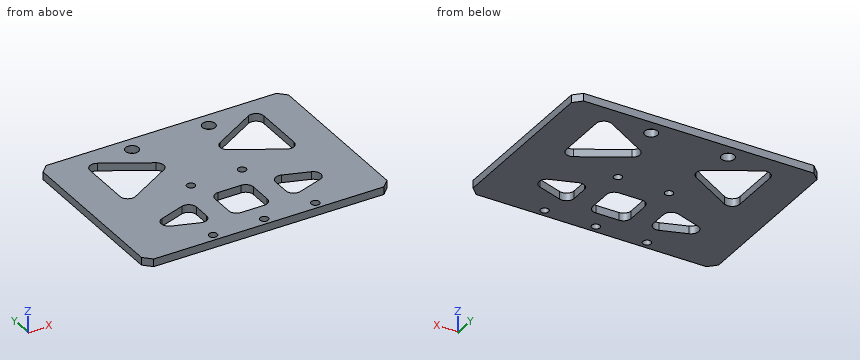
```python
from build123d import *

# Parameters (mm, degrees)
SKETCH_1_W           = 20
SKETCH_1_H           = 40
SKETCH_1_W_2         = 14
SKETCH_1_H_2         = 34
EXTRUDE_1_DEPTH      = 321
SKETCH_15_R          = 2.525
CUT_EXTRUDE_12_DEPTH = 21
SKETCH_18_W          = 17
SKETCH_18_H          = 40
CUT_EXTRUDE_14_DEPTH = 322
SKETCH_19_W          = 96
SKETCH_19_H          = 30
EXTRUDE_2_DEPTH      = 3
SKETCH_17_R          = 1.6
CUT_EXTRUDE_13_DEPTH = 4
FILLET_1_R           = 2
CHAMFER_1_SIZE       = 3
SKETCH_20_W          = 11
SKETCH_20_H          = 22.5
SKETCH_20_W_2        = 15
SKETCH_20_H_2        = 15
CUT_EXTRUDE_15_DEPTH = 4
FILLET_2_R           = 3
CUT_EXTRUDE_16_DEPTH = 4
FILLET_3_R           = 2
SKETCH_22_R          = 1.6
CUT_EXTRUDE_17_DEPTH = 4
CUT_EXTRUDE_19_DEPTH = 10
CHAMFER_2_SIZE       = 3
EXTRUDE_3_DEPTH      = 3
CUT_EXTRUDE_20_DEPTH = 4
FILLET_4_R           = 3


with BuildPart() as part:
    # 草图1 → 凸台-拉伸1 (new body)
    with BuildSketch(Plane(origin=(0, 0, 0), x_dir=(0, 0, -1), z_dir=(1, 0, 0))):
        Rectangle(SKETCH_1_W, SKETCH_1_H)
        Rectangle(SKETCH_1_W_2, SKETCH_1_H_2, mode=Mode.SUBTRACT)
    extrude(amount=EXTRUDE_1_DEPTH)

    # 草图15 → 切除-拉伸12 (cut, through all)
    with BuildSketch(Plane.XY.offset(10)):
        with Locations((145.5, 14)):
            Circle(SKETCH_15_R)
        with Locations((175.5, 14)):
            Circle(SKETCH_15_R)
    extrude(amount=-CUT_EXTRUDE_12_DEPTH, mode=Mode.SUBTRACT)

    # 草图18 → 切除-拉伸14 (cut, through all)
    with BuildSketch(Plane(origin=(321, 0, 0), x_dir=(0, 0, -1), z_dir=(1, 0, 0))):
        with Locations((1.5, 0)):
            Rectangle(SKETCH_18_W, SKETCH_18_H)
    extrude(amount=-CUT_EXTRUDE_14_DEPTH, mode=Mode.SUBTRACT)

    # 草图19 → 凸台-拉伸2 (add)
    with BuildSketch(Plane.XY.offset(10)):
        with Locations((160.5, -35)):
            Rectangle(SKETCH_19_W, SKETCH_19_H)
    extrude(amount=-EXTRUDE_2_DEPTH)

    # 草图17 → 切除-拉伸13 (cut, through all)
    with BuildSketch(Plane.XY.offset(10)):
        with Locations((12, 16.5)):
            Circle(SKETCH_17_R)
        with Locations((29, 16.5)):
            Circle(SKETCH_17_R)
        with Locations((12, -14)):
            Circle(SKETCH_17_R)
        with Locations((29, -14)):
            Circle(SKETCH_17_R)
        with Locations((43.5, -14)):
            Circle(SKETCH_17_R)
        with Locations((67.5, -14)):
            Circle(SKETCH_17_R)
        with Locations((222, -14)):
            Circle(SKETCH_17_R)
        with Locations((239, -14)):
            Circle(SKETCH_17_R)
        with Locations((253.5, -14)):
            Circle(SKETCH_17_R)
        with Locations((277.5, -14)):
            Circle(SKETCH_17_R)
        with Locations((292, -14)):
            Circle(SKETCH_17_R)
        with Locations((309, -14)):
            Circle(SKETCH_17_R)
        with Locations((82, -14)):
            Circle(SKETCH_17_R)
        with Locations((99, -14)):
            Circle(SKETCH_17_R)
        with Locations((292, 16.5)):
            Circle(SKETCH_17_R)
        with Locations((309, 16.5)):
            Circle(SKETCH_17_R)
        with Locations((140.5, -47)):
            Circle(SKETCH_17_R)
        with Locations((160.5, -47)):
            Circle(SKETCH_17_R)
        with Locations((180.5, -47)):
            Circle(SKETCH_17_R)
    extrude(amount=-CUT_EXTRUDE_13_DEPTH, mode=Mode.SUBTRACT)

    # 圆角1
    fillet_1_edges = [part.edges().sort_by_distance(p)[0] for p in [
        (208.5, -20, 8.5),
        (112.5, -20, 8.5),
    ]]
    fillet(fillet_1_edges, radius=FILLET_1_R)

    # 倒角1
    chamfer_1_edges = [part.edges().sort_by_distance(p)[0] for p in [
        (0, 20, 8.5),
        (321, 20, 8.5),
        (0, -20, 8.5),
        (208.5, -50, 8.5),
        (112.5, -50, 8.5),
        (321, -20, 8.5),
    ]]
    chamfer(chamfer_1_edges, length=CHAMFER_1_SIZE)

    # 草图20 → 切除-拉伸15 (cut, through all)
    with BuildSketch(Plane.XY.offset(10)):
        with Locations((300.5, 1.25)):
            Rectangle(SKETCH_20_W, SKETCH_20_H)
        with Locations((20.5, 1.25)):
            Rectangle(SKETCH_20_W, SKETCH_20_H)
        with Locations((160.5, -32)):
            Rectangle(SKETCH_20_W_2, SKETCH_20_H_2)
        Polygon((123, -32), (145, -24.5), (145, -39.5), align=None)
        Polygon((176, -24.5), (176, -39.5), (198, -32), align=None)
    extrude(amount=-CUT_EXTRUDE_15_DEPTH, mode=Mode.SUBTRACT)

    # 圆角2
    fillet_2_edges = [part.edges().sort_by_distance(p)[0] for p in [
        (26, 12.5, 8.5),
        (26, -10, 8.5),
        (15, -10, 8.5),
        (15, 12.5, 8.5),
        (176, -24.5, 8.5),
        (198, -32, 8.5),
        (176, -39.5, 8.5),
        (145, -39.5, 8.5),
        (123, -32, 8.5),
        (145, -24.5, 8.5),
        (168, -24.5, 8.5),
        (168, -39.5, 8.5),
        (153, -39.5, 8.5),
        (153, -24.5, 8.5),
        (306, 12.5, 8.5),
        (306, -10, 8.5),
        (295, -10, 8.5),
        (295, 12.5, 8.5),
    ]]
    fillet(fillet_2_edges, radius=FILLET_2_R)

    # 草图21 → 切除-拉伸16 (cut, through all)
    with BuildSketch(Plane.XY.offset(10)):
        Polygon((33, 6.144919815), (33, -10), (55.199264746, -10), align=None)
        Polygon((181.103828979, -10), (139.896171021, -10), (160.5, 8.609910045), align=None)
        Polygon((67.248892355, -8.871386982), (41.300735254, 10), (88.479202711, 10), align=None)
        Polygon((288, -10), (265.800735254, -10), (288, 6.144919815), align=None)
        Polygon((253.751107645, -8.871386982), (232.520797289, 10), (279.699264746, 10), align=None)
    extrude(amount=-CUT_EXTRUDE_16_DEPTH, mode=Mode.SUBTRACT)

    # 圆角3
    fillet_3_edges = [part.edges().sort_by_distance(p)[0] for p in [
        (279.699264746, 10, 8.5),
        (253.751107645, -8.871386982, 8.5),
        (232.520797289, 10, 8.5),
        (265.800735254, -10, 8.5),
        (288, 6.144919815, 8.5),
        (288, -10, 8.5),
        (160.5, 8.609910045, 8.5),
        (181.103828979, -10, 8.5),
        (139.896171021, -10, 8.5),
        (88.479202711, 10, 8.5),
        (67.248892355, -8.871386982, 8.5),
        (41.300735254, 10, 8.5),
        (33, 6.144919815, 8.5),
        (55.199264746, -10, 8.5),
        (33, -10, 8.5),
    ]]
    fillet(fillet_3_edges, radius=FILLET_3_R)

    # 草图22 → 切除-拉伸17 (cut, through all)
    with BuildSketch(Plane.XY.offset(10)):
        with Locations((150.5, -16)):
            Circle(SKETCH_22_R)
        with Locations((170.5, -16)):
            Circle(SKETCH_22_R)
    extrude(amount=-CUT_EXTRUDE_17_DEPTH, mode=Mode.SUBTRACT)

    # 草图26 → 切除-拉伸19 (cut)
    with BuildSketch(Plane.XY.offset(10)):
        with BuildLine():
            ThreePointArc((110.5, -20), (111.914213562, -20.585786438), (112.5, -22))
            Line((112.5, -22), (112.5, 20))
            Line((112.5, 20), (3, 20))
            Line((3, 20), (0, 17))
            Line((0, 17), (0, -17))
            Line((0, -17), (3, -20))
            Line((3, -20), (110.5, -20))
        make_face()
        with BuildLine():
            ThreePointArc((210.5, -20), (209.085786438, -20.585786438), (208.5, -22))
            Line((208.5, -22), (208.5, 20))
            Line((208.5, 20), (318, 20))
            Line((318, 20), (321, 17))
            Line((321, 17), (321, -17))
            Line((321, -17), (318, -20))
            Line((318, -20), (210.5, -20))
        make_face()
    extrude(amount=-CUT_EXTRUDE_19_DEPTH, mode=Mode.SUBTRACT)

    # 倒角2
    chamfer_2_edges = [part.edges().sort_by_distance(p)[0] for p in [
        (112.5, 20, 8.5),
        (208.5, 20, 8.5),
    ]]
    chamfer(chamfer_2_edges, length=CHAMFER_2_SIZE)

    # 草图27 → 凸台-拉伸3 (add)
    with BuildSketch(Plane.XY.offset(10)):
        with BuildLine():
            Line((145.094256532, -10), (175.905743468, -10))
            ThreePointArc((175.905743468, -10), (177.772346073, -8.718188495), (177.246315984, -6.515794714))
            Line((177.246315984, -6.515794714), (161.840572516, 7.399070354))
            ThreePointArc((161.840572516, 7.399070354), (160.5, 7.914865068), (159.159427484, 7.399070354))
            Line((159.159427484, 7.399070354), (143.753684016, -6.515794714))
            ThreePointArc((143.753684016, -6.515794714), (143.227653927, -8.718188495), (145.094256532, -10))
        make_face()
    extrude(amount=-EXTRUDE_3_DEPTH)

    # 草图28 → 切除-拉伸20 (cut, through all)
    with BuildSketch(Plane.XY.offset(10)):
        Polygon((126.519237886, 15), (152.5, 0), (126.519237886, -15), align=None)
        Polygon((168.5, 0), (194.480762114, -15), (194.480762114, 15), align=None)
    extrude(amount=-CUT_EXTRUDE_20_DEPTH, mode=Mode.SUBTRACT)

    # 圆角4
    fillet_4_edges = [part.edges().sort_by_distance(p)[0] for p in [
        (126.519237886, -15, 8.5),
        (126.519237886, 15, 8.5),
        (152.5, 0, 8.5),
        (168.5, 0, 8.5),
        (194.480762114, 15, 8.5),
        (194.480762114, -15, 8.5),
    ]]
    fillet(fillet_4_edges, radius=FILLET_4_R)


solid = part.part
```
Check sheet for the modelled part. Datum: model origin and axes. Units: mm. Give positions to 0.01 mm unless a question says otherwise; leave off trailing zeros. Loops run counter-clockwise (first coordinate to the right, second up) from the corner with the lowest first, then second, coordinate; pieces in that order, holes last. Notation, with made-up numbers: (-2, 70) - (12, 70) arc R30 ccw to (12, 100) - close; hole circle Ø4 at (-35.75, 28). An arc over 180 degrees is marked (long way). One line per question, with ' | ' between items. Start each with the question number.
1. Cross-section at C-C, the plane x = 187. Enter the section's corners in (y, z), plus the area to 3 significant figures.
2. Material ranges on line 1 along X through (y, z) = (-32, 8.95); line 2 along Y through (x, z) = (142.5, 8.7); line 3 along Y through (x, z) = (175.5, 8.5) (3 decimals), recorded low to high. Write a range as [from, to].
3. Cross-section at D-D, the plane z = 9.4. Give the number of separate pieces and of enclosed holes in the cut face, plus the area to 3 significant figures.
4. Cross-section at A-A, the plane y = -16. Enter the section's corners in (x, z).
5. Cross-section at B-B, the plane x = 170.5. Enter the section's corners in (y, z).
Check result:
1) outline: (-50, 7) - (-35.75, 7) - (-35.75, 10) - (-50, 10) - close; (-28.25, 7) - (-10.68, 7) - (-10.68, 10) - (-28.25, 10) - close; (10.68, 7) - (20, 7) - (20, 10) - (10.68, 10) - close | area: 123 mm2
2) line 1: x = [112.5, 129.3], [145, 153], [168, 176], [191.7, 208.5] | line 2: y = [-50, -38.27], [-25.73, -5.77], [5.77, 20] | line 3: y = [-50, -4.041], [4.041, 11.475], [16.525, 20]
3) separate pieces: 1 | enclosed holes: 12 | area: 5,380 mm2
4) outline: (112.5, 7) - (148.9, 7) - (148.9, 10) - (112.5, 10) - close; (152.1, 7) - (168.9, 7) - (168.9, 10) - (152.1, 10) - close; (172.1, 7) - (208.5, 7) - (208.5, 10) - (172.1, 10) - close
5) outline: (-50, 7) - (-17.6, 7) - (-17.6, 10) - (-50, 10) - close; (-14.4, 7) - (20, 7) - (20, 10) - (-14.4, 10) - close
